Check sheet for the drawn part. Datum: minimum x, y, z corner. Units: mm. A direction names the side the tool comes from. Give positions to 0.01 mm unless a question says otherwise; leave off trailing zeros. Loops run counter-clockwise (first coordinate to the right, second up) from the corner with the lowest first, then second, coordinate; pieces in that order, holes last.
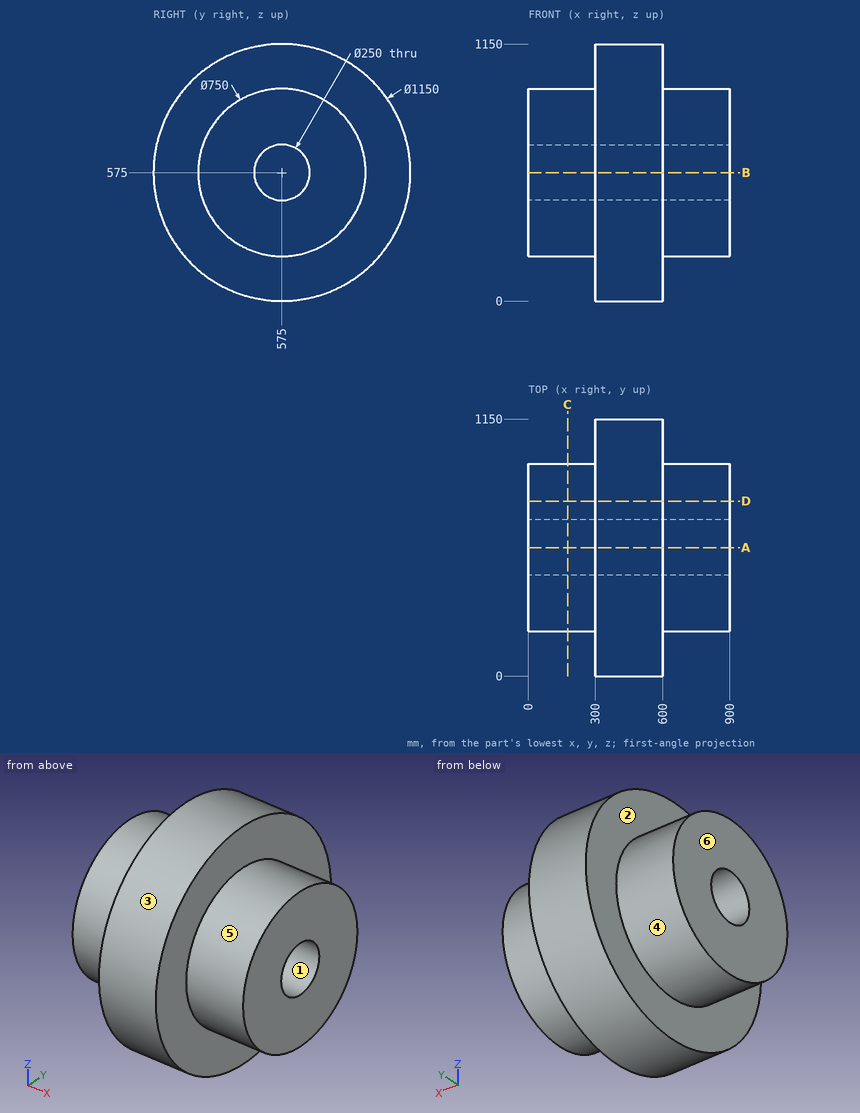
1) Sectioned sample at C-C on x = 175.5. Enter the section's corners in (y, z), plus the area to 3 significant figures.
2) Sectioned sample at D-D on y = 782. Enter the section's corners in (x, z), plus the area to 3 significant figures.
3) Scan lines: line 1 along Z through (x, y) = (700.5, 575); line 2 along Y through (x, z) = (576, 575). Record each from-to range of solid material in increasing order.
4) Sectioned sample at A-A on y = 575. Enter the section's corners in (x, z).
5) Mould release check, pull along Y, two halves, no side actions. Record for the marked faces 1, 2 and 3: +Y half, -Y half, draft (parallel to the pull), parting line (faces both ways), or undercut.
6) Depth check by flat-ended pin: P1, Ø4, axis at y = 241.5, z = 237, coming from the -X side; P2, Ø1, axis at x = 445, z = 408.5, coming from the +Y side; P3, Ø1.5, axis at y = 871, z = 210.5, coming from the +X side. Enter the tip coordinate at first touch or a pass-through.
7) Tool access check on the marked faces 4, 5 and 6. Record the directions out of +Z, -Z, +X, -X, +Y, -Y that give a thin tool (end or side, any length) a straight path to the whole face; none if there is none.
Determined:
1. outline: circle Ø750 at (575, 575); hole circle Ø250 at (575, 575)
1. area: 393,000 mm2
2. outline: (0, 262.31) - (300, 262.31) - (300, 38.55) - (600, 38.55) - (600, 262.31) - (900, 262.31) - (900, 887.69) - (600, 887.69) - (600, 1111.45) - (300, 1111.45) - (300, 887.69) - (0, 887.69) - close
2. area: 697,000 mm2
3. line 1: z = 200 to 450, 700 to 950
3. line 2: y = 0 to 450, 700 to 1150
4. outline: (0, 200) - (300, 200) - (300, 0) - (600, 0) - (600, 200) - (900, 200) - (900, 450) - (0, 450) - close; (0, 700) - (900, 700) - (900, 950) - (600, 950) - (600, 1150) - (300, 1150) - (300, 950) - (0, 950) - close
5. face 1: undercut
5. face 2: draft
5. face 3: parting line
6. P1: stops at x = 300
6. P2: stops at y = 1125.52
6. P3: stops at x = 600
7. face 4: -X
7. face 5: +X
7. face 6: +Z, -Z, -X, +Y, -Y
